Geometry: see drawing. Coordinates: mm, zero at the bounding-box minimum. A direction names the side the tool comes from. Give positions to 0.01 mm unless a question says otherwise; leave off trailing zeros. Write each loop counter-clockwise with the first axis right and the second up, starting at its lowest first coordinate (ties: lowest second). Pieces come first, ordered by that corner, then holes. Notation, with made-up numbers: (72, 87) -> (94, 87) arc R25 cw to (94, 121) -> close; hole circle Ø10 at (60.25, -4). An arc over 180 degrees is marked (long way). Answer as a JSON object with one key per item and string values. Group by question number.
Item 1: Section query D-D on x = 13.5. Return the cut outline in (y, z), plus the area to 3 significant figures.
Item 2: Section query A-A on z = 18.5. Return the cut outline in (x, y).
Item 3: Pull-direction query (Y, two-part tool) for the marked faces 4, 5 and 6; classes: pulls with the +Y half, pulls with the -Y half, needs draft (parallel to the pull), parting line crosses it, or undercut.
Item 4: Ray query, probe 1 along Y at (x, z) = (14, 26); probe 2 along X at (y, z) = (3.5, 13); probe 3 along X at (y, z) = (3.25, 20.25). Return the intervals inside material, ascending. Write a range as from..to.
Item 5: Section query C-C on z = 2. Return the cut outline in (x, y), plus the area to 3 significant figures.
Item 6: Access query for the marked faces 1, 2 and 3. Directions: +Z, -Z, +X, -X, +Y, -Y. A direction counts if a zero-diameter tool reaches every point of the face in a straight line with its end or side. Return the directions, or none.
Item 7: First-contact query: pin 1 Ø10 at (x, z) = (6, 19.5) entering from -Y; pin 2 Ø3 at (y, z) = (1.5, 25) entering from -X; pin 3 Ø5 at (x, z) = (15.5, 10) entering from +Y; pin 4 Ø4 at (x, y) = (3.5, 6) entering from +Z. Flat tips, straight axial feed; report the tip coordinate or a pass-through.
Item 8: Section query B-B on x = 5. Return the cut outline in (y, z).
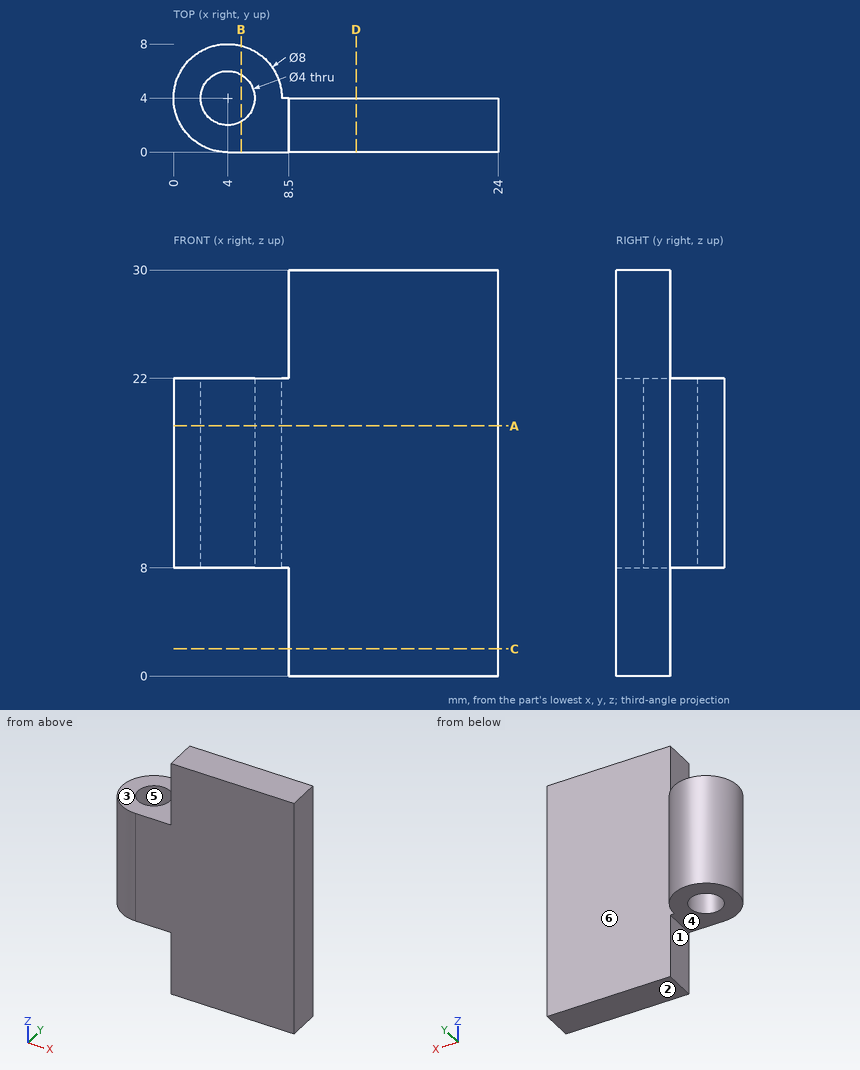
Worked answers:
{
 "1": {"outline": "(0, 0) -> (4, 0) -> (4, 30) -> (0, 30) -> close", "area": "120 mm^2"},
 "2": {"outline": "(4, 0) -> (24, 0) -> (24, 4) -> (8, 4) arc R4 ccw (long way) to start; hole circle Ø4 at (4, 4)"},
 "3": {"face 4": "needs draft", "face 5": "undercut", "face 6": "pulls with the +Y half"},
 "4": {"probe 1": "0..4", "probe 2": "0.03..2.06, 5.94..24", "probe 3": "0.07..2.15, 5.85..24"},
 "5": {"outline": "(8.5, 0) -> (24, 0) -> (24, 4) -> (8.5, 4) -> close", "area": "62.0 mm^2"},
 "6": {"face 1": "-Z, -X, +Y, -Y", "face 2": "-Z, +X, -X, +Y, -Y", "face 3": "+Z, -X, +Y, -Y"},
 "7": {"pin 1": "y = 0", "pin 2": "x = 8.5", "pin 3": "y = 4", "pin 4": "z = 22"},
 "8": {"outline": "(0, 8) -> (2.27, 8) -> (2.27, 22) -> (0, 22) -> close; (5.73, 8) -> (7.87, 8) -> (7.87, 22) -> (5.73, 22) -> close"}
}
